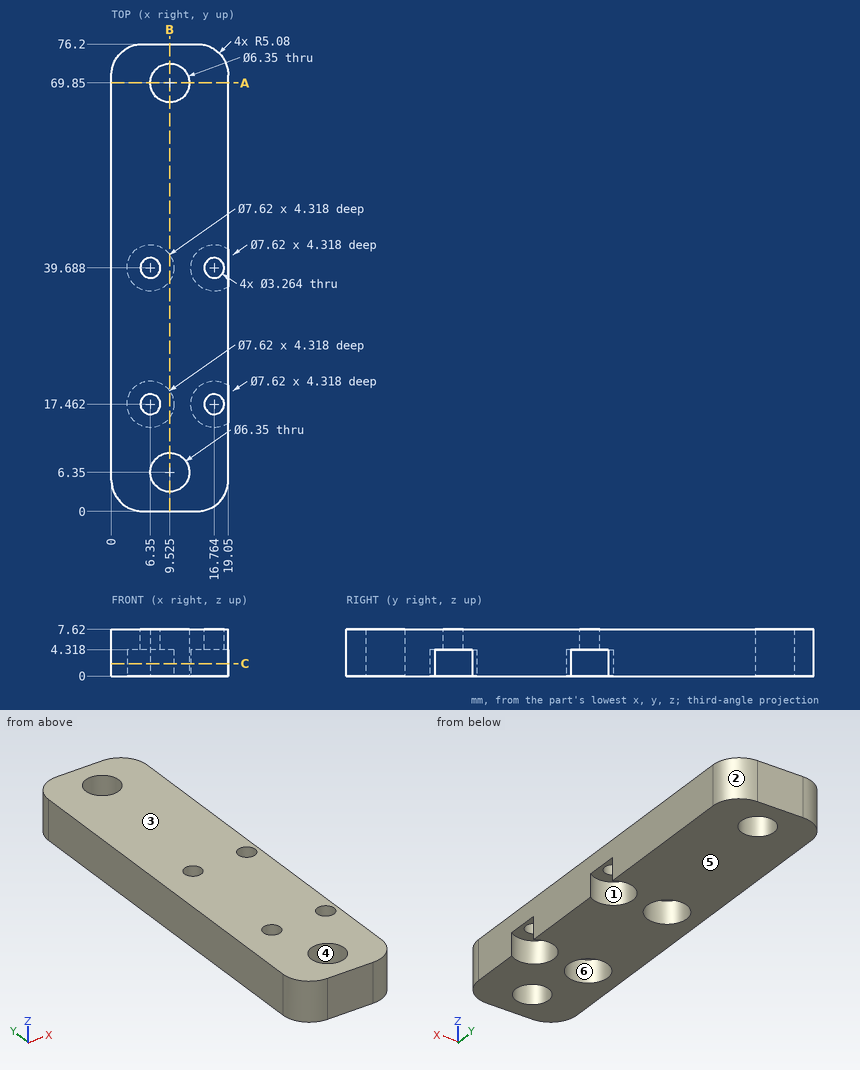
Job drawing, mm, ordinate dimensions from the low corner. One solid piece. A direction names the side the tool comes from. Give positions to 0.01 mm unless a question says otherwise; leave off trailing zeros. Write each loop counter-clockwise with the first axis right and the second up, starting at its lowest first coordinate (ties: lowest second). Pieces come first, ordered by that corner, then holes. Notation, with made-up numbers: (36.25, 60.25) - (67.25, 60.25) arc R16 cw to (67.25, 79.25) - close; hole circle Ø4 at (50.25, -12). An arc over 180 degrees is marked (long way). Answer as CSV lines item,"result".
1. Drill centre lines: L1, parallel to X at y = 39.5, z = 1.25 (1 decimal); L2, parallel to Y at x = 17.25, z = 1 (1 decimal); L3, parallel to Y at x = 12, z = 2.75. Where is each one in solid material? Low to high. Write a range as [from, to].
Responses:
L1,"x = [0, 2.5], [10.2, 13]"
L2,"y = [1.2, 13.7], [21.2, 35.9], [43.5, 75]"
L3,"y = [0, 4.36], [8.34, 67.86], [71.84, 76.2]"
2. Two-plate mould, pull along X, no slides. Class the marked faces 1, 2, 3 and 4: +X half, -X half, draft (parallel to the pull), parting line (faces both ways), or undercut.
Responses:
face 1,"undercut"
face 2,"+X half"
face 3,"draft"
face 4,"undercut"
3. 3-axis set-ups, long thin cutter, end or side, ignore diameter. For the marked faces 5 and 6: which of +Z, -Z, +X, -X, +Y, -Y reach the whole face in a straight line?
Responses:
face 5,"-Z, +X, -X, +Y, -Y"
face 6,"-Z"
4. Band-saw the part on B-B (x = 9.5). Write the cut outline in (y, z) (1 decimal).
Responses:
outline,"(0, 0) - (3.2, 0) - (3.2, 7.6) - (0, 7.6) - close; (9.5, 0) - (15.3, 0) - (15.3, 4.3) - (19.6, 4.3) - (19.6, 0) - (37.5, 0) - (37.5, 4.3) - (41.8, 4.3) - (41.8, 0) - (66.7, 0) - (66.7, 7.6) - (9.5, 7.6) - close; (73, 0) - (76.2, 0) - (76.2, 7.6) - (73, 7.6) - close"
5. Pin check, flat tip, straight feed: pin 1 (5 mm diameter, centred on x = 16.76, y = 17.46, fed in from -Z). Stop position of the tip, or through.
Responses:
pin 1,"stops at z = 4.32"
6. Band-saw the part on A-A (y = 69.85). Write the cut outline in (x, z).
Responses:
outline,"(0, 0) - (6.35, 0) - (6.35, 7.62) - (0, 7.62) - close; (12.7, 0) - (19.05, 0) - (19.05, 7.62) - (12.7, 7.62) - close"
7. Band-saw the part on C-C (z = 2). Count the separate pieces of the cut face and the enclosed holes in it, and give its area (3 significant figures).
Responses:
separate pieces,"1"
enclosed holes,"4"
area,"1,200 mm2"
